```python
from build123d import *

# Parameters (mm, degrees)
F1_DEPTH = 12.7
F2_R     = 6.34999
F3_R     = 6.34999
F4_DEPTH = 3.175
F6_D     = 4.826
F6_DEPTH = 14.224
F6_TIP   = 1.4498766737
F8_D     = 4.826
F8_DEPTH = 14.224
F8_TIP   = 1.4498766737


# Not quite as in the source:
# - a fillet or chamfer is up to 0.001 mm smaller than in the source, because OpenCascade refuses the exact size


with BuildPart() as f1:
    # F0 (on Front) → F1 (new body)
    with BuildSketch(Plane.XZ):
        Polygon((12.7, 64.008), (12.7, 68.2625), (-12.7, 68.2625), (-12.7, -68.2625), (12.7, -68.2625), (12.7, -64.008), (12.7, -58.7375), (0, -58.7375), (0, 58.7375), (12.7, 58.7375), align=None)
    extrude(amount=F1_DEPTH)

    # F2 (radius 6.35 in the source; OpenCascade refuses exactly that, so slightly less here)
    f2_edges = [f1.edges().sort_by_distance(p)[0] for p in [
        (0, -12.7, 0),
        (0, 0, 0),
    ]]
    fillet(f2_edges, radius=F2_R)

    # F3 (radius 6.35 in the source; OpenCascade refuses exactly that, so slightly less here)
    f3_edges = [f1.edges().sort_by_distance(p)[0] for p in [
        (6.35, -12.7, 58.7375),
        (6.35, 0, 58.7375),
        (6.35, -12.7, -58.7375),
        (6.35, 0, -58.7375),
    ]]
    fillet(f3_edges, radius=F3_R)

    # F4 (cut): a face of the model
    f4_faces = [f1.faces().sort_by_distance(p)[0] for p in [
        (-12.7, -6.35, 0),
    ]]
    extrude(f4_faces, amount=-F4_DEPTH, mode=Mode.SUBTRACT)

    # F6
    with Locations(Plane.YZ.offset(12.7)):
        with Locations((-6.35, 63.1825)):
            Hole(F6_D / 2, depth=F6_DEPTH)
            with Locations((0, 0, -(F6_DEPTH + F6_TIP / 2))):  # 118° drill point
                Cone(0, F6_D / 2, F6_TIP, mode=Mode.SUBTRACT)

    # F8
    with Locations(Plane.YZ.offset(12.7)):
        with Locations((-6.35, -64.008)):
            Hole(F8_D / 2, depth=F8_DEPTH)
            with Locations((0, 0, -(F8_DEPTH + F8_TIP / 2))):  # 118° drill point
                Cone(0, F8_D / 2, F8_TIP, mode=Mode.SUBTRACT)


solid = f1.part
```
The model under review builds one solid part; all positions refer to its coordinate system, in mm. A direction names the side the tool comes from. Round coordinates to 2 decimals unless told otherwise and drop trailing zeros. Order: outer loops, then holes, each group sorted by start corner. A loop starts at its lowest first (then second) coordinate and runs counter-clockwise, first axis right, second up. Notation, with made-up numbers: (25.5, -35.75) -> (52.5, -35.75) arc R29 ccw to (52.5, -10.75) -> close; hole circle Ø5 at (76, 52.5). An arc over 180 degrees is marked (long way). One line per item, written item: value. Start each with the question number.
Q1. Mouldability with a two-part tool opening along Z and no side actions: class faces 4 (the face through (5.43, -10.79, 60.55)), 5 (the face through (12.7, -8, 66)), 6 (the face through (2, -6, 68.262)) as released by +Z, released by -Z, zero draft, split by the parting line, or undercut.
Q2. Wall thickness on line 1 (Z direction, x = 2, y = -6.35) (1 decimal); line 2 (Z direction, x = 8.5, y = -8); line 3 (Y direction, x = -5.75, z = -21): over which ranges is each line inside the solid? List them lowest first.
Q3. Take a section at C-C (y = -10.5). Write out the cut boundary in (x, z) (1 decimal).
Q4. Clearance check with flat-ended pins moving along their axes: pin 1 Ø3 at (y, z) = (-6.35, 63.18) entering from +X; pin 2 Ø1.5 at (x, z) = (-4, 16) entering from -Y; pin 3 Ø1.5 at (y, z) = (-10.5, -42.5) entering from +X. State where each tip first meets the part, or that it passes through.
Q5. Take a section at A-A (x = 8). Count the separate pieces of the cut face and the enclosed holes in it, and give its area (3 significant figures).
Q6. Machinability: for faces 1 (the face through (5.16, -1.91, 60.55)), 2 (the face through (5.49, -7.46, 61.04)), 3 (the face through (-1.81, -10.79, 0.91)), which of the approach directions +Z, -Z, +X, -X, +Y, -Y give a long, thin tool a straight path to every point of the face, cutting with its end or side? Answer none if there is none.
Reported:
1. face 4: undercut
1. face 5: zero draft
1. face 6: released by +Z
2. line 1: z = -68.3 to -66.4, -61.6 to -58.7, 58.7 to 60.8, 65.6 to 68.3
2. line 2: z = -68.26 to -65.77, -62.25 to -58.96, 58.96 to 61.42, 64.94 to 68.26
2. line 3: y = -12.67 to -0.03
3. outline: (-9.5, -68.3) -> (12.7, -68.3) -> (12.7, -60.3) -> (-1.5, -60.3) -> (-1.5, 60.3) -> (12.7, 60.3) -> (12.7, 68.3) -> (-9.5, 68.3) -> close
4. pin 1: stops at x = -2.07
4. pin 2: stops at y = -12.5
4. pin 3: stops at x = -0.99
5. separate pieces: 2
5. enclosed holes: 2
5. area: 171 mm2
6. face 1: +X, +Y
6. face 2: +X
6. face 3: +X, -Y
